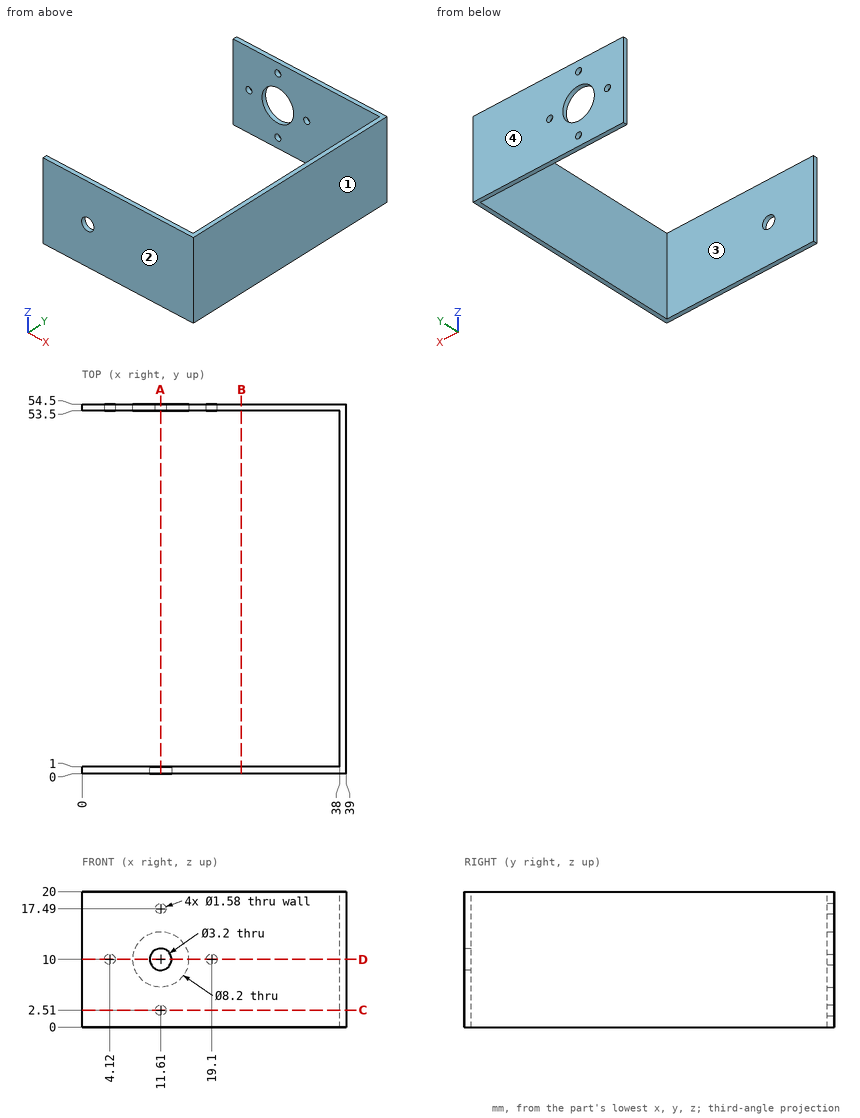
Study the drawing (mm; zero at the part's minimum x, y, z) and answer. Coordinates: 2 decimals unless noted, no trailing zeros. Loops run counter-clockwise (first coordinate to the right, second up) from the corner with the lowest first, then second, coordinate; pieces in that order, holes last. Notation, with made-up numbers: M 52.5,20.25 L 70.5,20.25 A18 ccw 70.5,33.25 Z; hole C -29.5,-23.5 d5. An arc over 180 degrees is marked long. Answer in a Markdown table with one row per item. Add a question column.
1. Flat-ended cylindrical pins translate along their axes: P1, Ø3.5, axis at x = 11.61, z = 10, coming from the +Y side; P2, Ø1.4, axis at x = 11.61, z = 17.49, coming from the -Y side; P3, Ø3, axis at y = 32, z = 8.5, coming from the -X side. Find the tip coordinate at first contact, or state that the pin passes through.
2. Find section D-D, the plane z = 10. Write down the section's boundary in (x, y), then the cut area to 3 significant figures.
3. Find section A-A, the plane x = 11.61. Write down the section's boundary in (y, z).
4. Find section B-B, the plane x = 23.5. Write down the section's boundary in (y, z), then the cut area to 3 significant figures.
5. Find section C-C, the plane z = 2.51. Write down the section's boundary in (x, y).
6. The mould has two halves that part along Y. Classify the marked faces 1, 2, 3 and 4: pulls with the +Y half, pulls with the -Y half, needs draft (parallel to the pull), parting line crosses it, or undercut.
7. Consider L1, parallel to Z at x = 11.61, y = 53.9; L2, parallel to X at y = 53.8, z = 10; L3, parallel to Y at x = 35, z = 4.25. Determine where each line is inside the solid, lowest interval first.
Reported:
| question | item | result |
|---|---|---|
| 1 | P1 | stops at y = 1 |
| 1 | P2 | stops at y = 0 |
| 1 | P3 | stops at x = 38 |
| 2 | outline | M 0,0 L 10.01,0 L 10.01,1 L 0,1 Z; M 0,53.5 L 3.33,53.5 L 3.33,54.5 L 0,54.5 Z; M 4.91,53.5 L 7.51,53.5 L 7.51,54.5 L 4.91,54.5 Z; M 13.21,0 L 39,0 L 39,54.5 L 19.89,54.5 L 19.89,53.5 L 38,53.5 L 38,1 L 13.21,1 Z; M 15.71,53.5 L 18.31,53.5 L 18.31,54.5 L 15.71,54.5 Z |
| 2 | area | 116 mm^2 |
| 3 | outline | M 0,0 L 1,0 L 1,8.4 L 0,8.4 Z; M 0,11.6 L 1,11.6 L 1,20 L 0,20 Z; M 53.5,0 L 54.5,0 L 54.5,1.72 L 53.5,1.72 Z; M 53.5,3.3 L 54.5,3.3 L 54.5,5.9 L 53.5,5.9 Z; M 53.5,14.1 L 54.5,14.1 L 54.5,16.7 L 53.5,16.7 Z; M 53.5,18.28 L 54.5,18.28 L 54.5,20 L 53.5,20 Z |
| 4 | outline | M 0,0 L 1,0 L 1,20 L 0,20 Z; M 53.5,0 L 54.5,0 L 54.5,20 L 53.5,20 Z |
| 4 | area | 40.0 mm^2 |
| 5 | outline | M 0,0 L 39,0 L 39,54.5 L 12.4,54.5 L 12.4,53.5 L 38,53.5 L 38,1 L 0,1 Z; M 0,53.5 L 10.82,53.5 L 10.82,54.5 L 0,54.5 Z |
| 6 | face 1 | needs draft |
| 6 | face 2 | pulls with the -Y half |
| 6 | face 3 | undercut |
| 6 | face 4 | pulls with the +Y half |
| 7 | L1 | z = 0 to 1.72, 3.3 to 5.9, 14.1 to 16.7, 18.28 to 20 |
| 7 | L2 | x = 0 to 3.33, 4.91 to 7.51, 15.71 to 18.31, 19.89 to 39 |
| 7 | L3 | y = 0 to 1, 53.5 to 54.5 |
